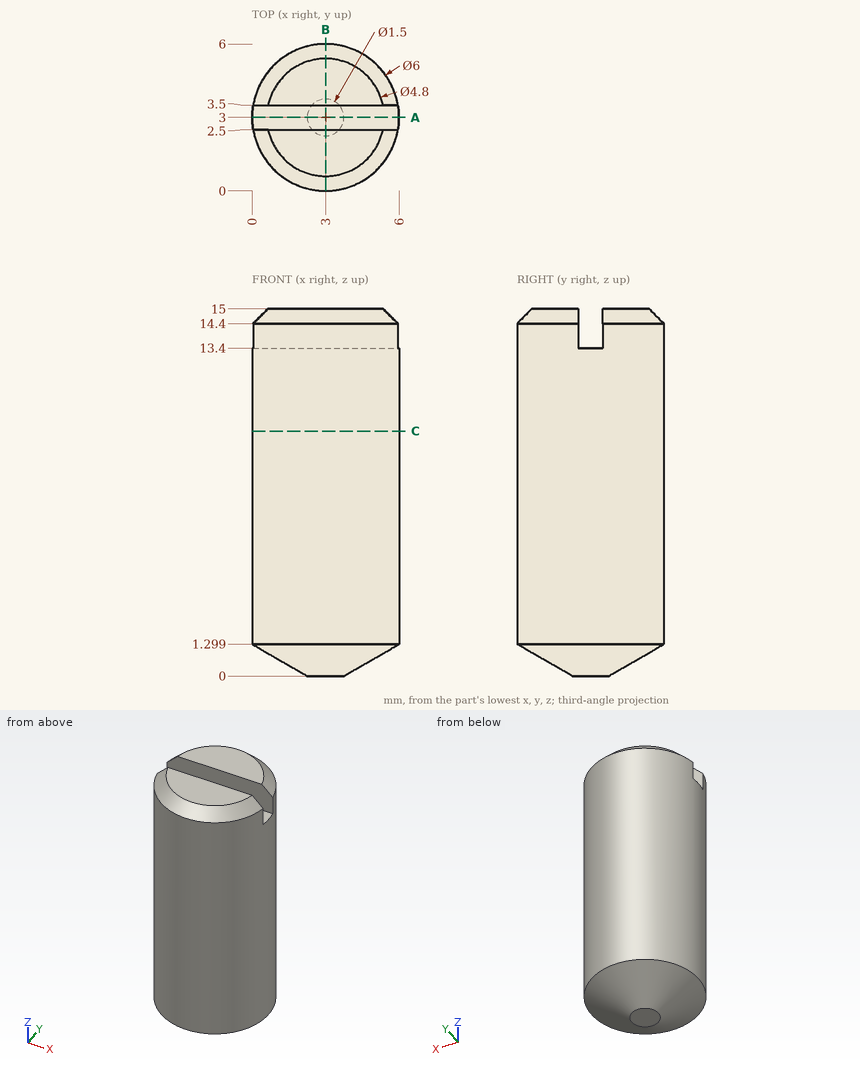
Answer from the drawing. Dimensions are ordinates in mm from the lowest x, y and z of the part. Round coordinates to 2 decimals unless told otherwise and drop trailing zeros. Loops run counter-clockwise (first coordinate to the right, second up) from the corner with the lowest first, then second, coordinate; pieces in that order, holes last.
Q1. Consider probe 1 along X at (y, z) = (4.8, 11.5); probe 2 along Z at (x, y) = (3.2, 2.85); probe 3 along Y at (x, z) = (1.65, 14). Determine where each line is inside the solid, lowest interval first.
Q2. Each of these flat-tipped pins is pushed along its axis until it touches: pin 1 (1.3 mm diameter, centred on x = 2, z = 14, fed in from +Y); pin 2 (2 mm diameter, centred on x = 2, y = 5, fed in from -Z); pin 3 (0.5 mm diameter, centred on x = 3.5, z = 14.5, fed in from -Y). Where does it stop, or does it pass through?
Q3. Section A-A on y = 3 is taken. Write down the section's boundary in (x, z).
Q4. Section B-B on x = 3 is taken. Write down the section's boundary in (y, z), and give its area (3 significant figures).
Q5. Section C-C on z = 10 is taken. Write down the section's boundary in (x, y), and give its area (3 significant figures).
Output:
1. probe 1: x = 0.6 to 5.4
1. probe 2: z = 0 to 13.4
1. probe 3: y = 0.32 to 2.5, 3.5 to 5.68
2. pin 1: stops at y = 5.98
2. pin 2: stops at z = 0.28
2. pin 3: stops at y = 0.01
3. outline: (0, 1.3) - (2.25, 0) - (3.75, 0) - (6, 1.3) - (6, 13.4) - (0, 13.4) - close
4. outline: (0, 1.3) - (2.25, 0) - (3.75, 0) - (6, 1.3) - (6, 14.4) - (5.4, 15) - (3.5, 15) - (3.5, 13.4) - (2.5, 13.4) - (2.5, 15) - (0.6, 15) - (0, 14.4) - close
4. area: 85.1 mm2
5. outline: circle Ø6 at (3, 3)
5. area: 28.3 mm2
